Job drawing, mm, ordinate dimensions from the low corner. One solid piece. A direction names the side the tool comes from. Give positions to 0.01 mm unless a question says otherwise; leave off trailing zeros. Loops run counter-clockwise (first coordinate to the right, second up) from the corner with the lowest first, then second, coordinate; pieces in that order, holes last. Notation, with made-up numbers: (-39, -37.5) - (15, -37.5) arc R26 ccw to (15, -23.5) - close; hole circle Ø7 at (4, -13.75). An arc over 180 degrees is marked (long way). Use a Markdown table: item, result.
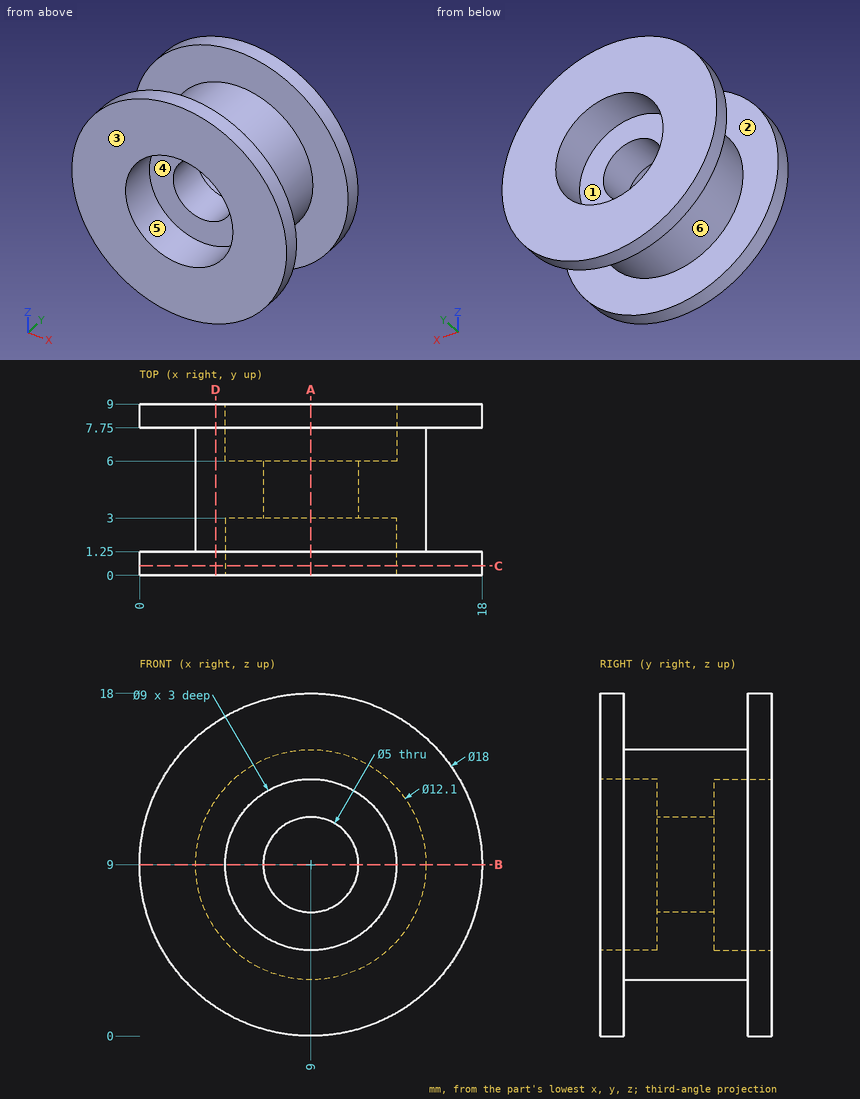
(1) Slice it at B-B, the plane z = 9. Write the cut outline in (x, y).
Computed:
| item | result |
|---|---|
| outline | (0, 0) - (4.5, 0) - (4.5, 3) - (6.5, 3) - (6.5, 6) - (4.5, 6) - (4.5, 9) - (0, 9) - (0, 7.75) - (2.95, 7.75) - (2.95, 1.25) - (0, 1.25) - close; (11.5, 3) - (13.5, 3) - (13.5, 0) - (18, 0) - (18, 1.25) - (15.05, 1.25) - (15.05, 7.75) - (18, 7.75) - (18, 9) - (13.5, 9) - (13.5, 6) - (11.5, 6) - close |
(2) Slice it at D-D, the plane x = 4. Write the cut outline in (y, z), plus the area to 3 significant figures.
Computed:
| item | result |
|---|---|
| outline | (0, 1.52) - (1.25, 1.52) - (1.25, 5.59) - (7.75, 5.59) - (7.75, 1.52) - (9, 1.52) - (9, 16.48) - (7.75, 16.48) - (7.75, 12.41) - (1.25, 12.41) - (1.25, 16.48) - (0, 16.48) - close |
| area | 81.7 mm² |
(3) Slice it at C-C, the plane y = 0.5. Write the cut outline in (x, z).
Computed:
| item | result |
|---|---|
| outline | circle Ø18 at (9, 9); hole circle Ø9 at (9, 9) |
(4) Pin check, flat tips, straight feed: P1, Ø2, axis at y = 2, z = 2.5, coming from the +X side; P2, Ø10, axis at x = 5, z = 6.5, coming from the -Y side; P3, Ø6.5, axis at x = 9, z = 9, coming from the -Y side. Stop position of each tip, or through.
Computed:
| item | result |
|---|---|
| P1 | x = 15.85 |
| P2 | y = 0 |
| P3 | y = 3 |
(5) 3-axis set-ups, long thin cutter, end or side, ignore diameter. For the marked faces 1, 2 and 3: which of +Z, -Z, +X, -X, +Y, -Y reach the whole face in a straight line?
Computed:
| item | result |
|---|---|
| face 1 | +Y |
| face 2 | none |
| face 3 | +Z, -Z, +X, -X, -Y |
(6) Slice it at A-A, the plane x = 9. Write the cut outline in (y, z), plus the area to 4 significant figures.
Computed:
| item | result |
|---|---|
| outline | (0, 0) - (1.25, 0) - (1.25, 2.95) - (7.75, 2.95) - (7.75, 0) - (9, 0) - (9, 4.5) - (6, 4.5) - (6, 6.5) - (3, 6.5) - (3, 4.5) - (0, 4.5) - close; (0, 13.5) - (3, 13.5) - (3, 11.5) - (6, 11.5) - (6, 13.5) - (9, 13.5) - (9, 18) - (7.75, 18) - (7.75, 15.05) - (1.25, 15.05) - (1.25, 18) - (0, 18) - close |
| area | 54.65 mm² |
(7) Mould opens along Y. For the marked faces 4, 5 and 6 say: pulls with the +Y half, pulls with the -Y half, needs draft (parallel to the pull), parting line crosses it, or undercut.
Computed:
| item | result |
|---|---|
| face 4 | pulls with the -Y half |
| face 5 | needs draft |
| face 6 | undercut |
(8) Drill centre lines: probe 1 along Z at (x, y) = (9, 4.2); probe 2 along X at (y, z) = (6.7, 9); probe 3 along Y at (x, z) = (12.25, 3.75). Where is each one in solid material? Low to high. Write a range as [from, to].
Computed:
| item | result |
|---|---|
| probe 1 | [2.95, 6.5], [11.5, 15.05] |
| probe 2 | [2.95, 4.5], [13.5, 15.05] |
| probe 3 | [0, 1.25], [7.75, 9] |
